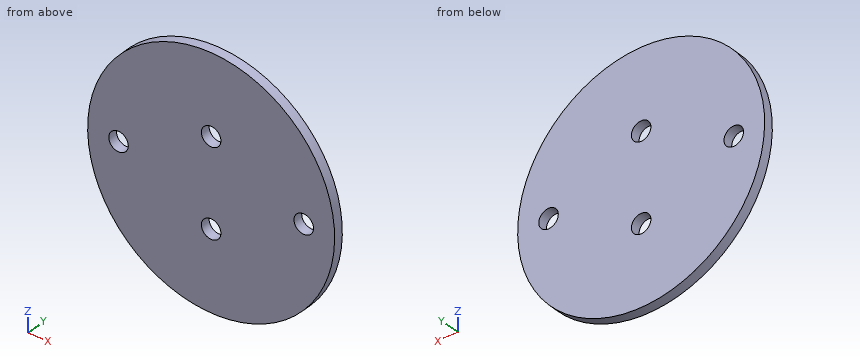
from build123d import *

# Parameters (mm, degrees)
SKETCH1_R           = 38
SKETCH1_R_2         = 3
BOSS_EXTRUDE1_DEPTH = 3


with BuildPart() as part:
    # Sketch1 → Boss-Extrude1 (new body)
    with BuildSketch(Plane(origin=(0, 0, 0), x_dir=(1, 0, 0), z_dir=(0, 1, 0))):
        with Locations(Location((0, 0, 0), (0, 0, 270))):
            Circle(SKETCH1_R)
        with Locations(Location((28.5, 0, 0), (0, 0, 270))):
            Circle(SKETCH1_R_2, mode=Mode.SUBTRACT)
        with Locations(Location((-28.5, 0, 0), (0, 0, 270))):
            Circle(SKETCH1_R_2, mode=Mode.SUBTRACT)
        with Locations(Location((0, 13.5, 0), (0, 0, 270))):
            Circle(SKETCH1_R_2, mode=Mode.SUBTRACT)
        with Locations(Location((0, -13.5, 0), (0, 0, 270))):
            Circle(SKETCH1_R_2, mode=Mode.SUBTRACT)
    extrude(amount=-BOSS_EXTRUDE1_DEPTH)


solid = part.part
The listing builds one solid part. Answer for the finished solid, in the listing's coordinates (mm). Give positions to 0.01 mm unless a question says otherwise; leave off trailing zeros. Loops run counter-clockwise (first coordinate to the right, second up) from the corner with the lowest first, then second, coordinate; pieces in that order, holes last. Notation, with made-up numbers: (-31.5, 20.25) - (24.5, 20.25) arc R15 cw to (24.5, 48.25) - close; hole circle Ø1 at (63, 73.5). An arc over 180 degrees is marked (long way). Use one line per item in the form item = value.
1. Section D-D on x = -28.5 is taken. Give the vertices of the cut face in (y, z).
Calculated:
outline = (-3, -25.13) - (0, -25.13) - (0, -3) - (-3, -3) - close; (-3, 3) - (0, 3) - (0, 25.13) - (-3, 25.13) - close
2. Section C-C on y = -1.8 is taken. Give the vertices of the cut face in (x, z).
Calculated:
outline = circle Ø76 at (0, 0); hole circle Ø6 at (-28.5, 0); hole circle Ø6 at (0, -13.5); hole circle Ø6 at (0, 13.5); hole circle Ø6 at (28.5, 0)
3. Section A-A on x = 0 is taken. Give the vertices of the cut face in (y, z), then the cut area to 3 significant figures.
Calculated:
outline = (-3, -38) - (0, -38) - (0, -16.5) - (-3, -16.5) - close; (-3, -10.5) - (0, -10.5) - (0, 10.5) - (-3, 10.5) - close; (-3, 16.5) - (0, 16.5) - (0, 38) - (-3, 38) - close
area = 192 mm^2
4. Given pin 1 Ø5 at (x, z) = (28.5, 0) entering from +Y; pin 2 Ø1 at (x, y) = (-7.5, -1) entering from -Z, each flat-ended and moving along its own axis, determine where each tip first touches the part or whether it passes through.
Calculated:
pin_1 = through
pin_2 = -37.35
5. Section B-B on z = 0 is taken. Give the vertices of the cut face in (x, y).
Calculated:
outline = (-38, -3) - (-31.5, -3) - (-31.5, 0) - (-38, 0) - close; (-25.5, -3) - (25.5, -3) - (25.5, 0) - (-25.5, 0) - close; (31.5, -3) - (38, -3) - (38, 0) - (31.5, 0) - close
6. Find the intervals of material crossed by line 1 along X through (y, z) = (-2.05, 0); line 2 along Z through (x, y) = (-0.5, -2.65); line 3 along Z through (x, y) = (-26.5, -1.25), in increasing order. Write a range as [from, to].
Calculated:
line_1 = [-38, -31.5], [-25.5, 25.5], [31.5, 38]
line_2 = [-38, -16.46], [-10.54, 10.54], [16.46, 38]
line_3 = [-27.24, -2.24], [2.24, 27.24]
